Can you work these out from the model? Positions are in its coordinate system, mm. Coordinates: 2 decimals unless noted, no trailing zeros. Loops run counter-clockwise (first coordinate to the right, second up) from the corner with the lowest first, then second, coordinate; pieces in that order, holes last. Notation, with made-up numbers: M 3.25,82.25 L 11.25,82.25 A9 cw 11.25,98.25 Z; hole C -21.75,55.5 d6. An arc over 180 degrees is marked long. Answer as a JSON object with one key per item and string values. Group by question number.
Item 1: Suppose I cut it at A-A (x = -82.55). Write out the boundary of the cut face in (y, z) (3 decimals), then the cut area to 3 significant figures.
Item 2: If I drill on line 1 (X direction, y = 152.4, z = 1.9) (3 decimals); line 2 (Y direction, x = -82.55, z = 1.95) (3 decimals); line 3 (Y direction, x = -27, z = 1.9), over which ranges is the centre line in solid material (lowest first)?
Item 3: Suppose I cut it at D-D (x = -67). Write out the boundary of the cut face in (y, z).
Item 4: Suppose I cut it at C-C (y = 43). Write out the boundary of the cut face in (x, z).
Item 5: I'm going to push a flat-ended pin straight in: pin 1 Ø1.5 at (x, z) = (-66, 0.5) entering from +Y. Where does the tip first touch, or does it pass through?
```python
from build123d import *

# Parameters (mm, degrees)
SKETCH1_R           = 3.175
BOSS_EXTRUDE1_DEPTH = 2.54


with BuildPart() as part:
    # Sketch1 → Boss-Extrude1 (new body)
    with BuildSketch(Plane.XY):
        with BuildLine():
            Line((0, 0), (-114.3, 0))
            Line((-114.3, 0), (-114.3, 152.4))
            ThreePointArc((-114.3, 152.4), (-82.55, 184.15), (-50.8, 152.4))
            ThreePointArc((-50.8, 152.4), (-48.798325541, 104.89333556), (-25.4, 63.5))
            Line((-25.4, 63.5), (-5.08, 17.582246738))
            ThreePointArc((-5.08, 17.582246738), (-9.150707628, 6.881106109), (0, 0))
        make_face()
        with Locations((-82.55, 152.4)):
            Circle(SKETCH1_R, mode=Mode.SUBTRACT)
    extrude(amount=BOSS_EXTRUDE1_DEPTH)


solid = part.part
```
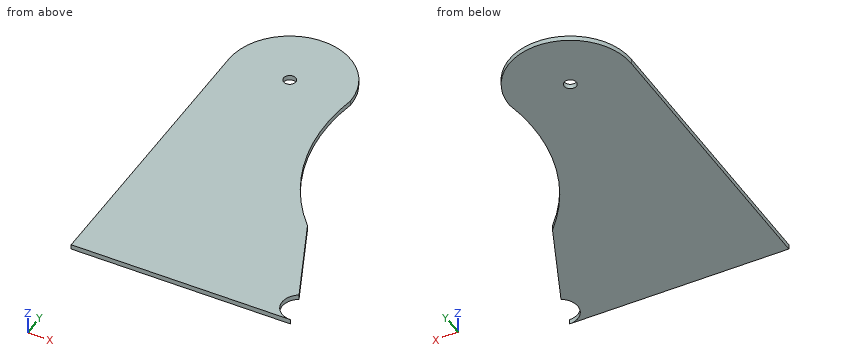
From the geometry:
{
 "1": {"outline": "M 0,0 L 149.225,0 L 149.225,2.54 L 0,2.54 Z; M 155.575,0 L 184.15,0 L 184.15,2.54 L 155.575,2.54 Z", "area": "452 mm2"},
 "2": {"line 1": "-114.3 to -85.725, -79.375 to -50.8", "line 2": "0 to 149.225, 155.575 to 184.15", "line 3": "0 to 65.26"},
 "3": {"outline": "M 0,0 L 180.08,0 L 180.08,2.54 L 0,2.54 Z"},
 "4": {"outline": "M -114.3,0 L -16.33,0 L -16.33,2.54 L -114.3,2.54 Z"},
 "5": {"pin 1": "y = 179.94"}
}
